Work out the finished part from the listing and answer in its coordinate system (mm). A direction names the side the tool comes from. Give positions to 0.01 mm unless a question says otherwise; leave off trailing zeros. Order: outer loops, then holes, each group sorted by start corner. A loop starts at its lowest first (then second) coordinate and runs counter-clockwise, first axis right, second up.
```python
from build123d import *

# Parameters (mm, degrees)
SKETCH1_W               = 50
SKETCH1_H               = 60
BOSS_EXTRUDE1_DEPTH     = 15
FILLET1_R               = 2
SKETCH2_W               = 40
SKETCH2_H               = 35
CUT_EXTRUDE1_DEPTH      = 6
SKETCH3_W               = 4
SKETCH3_H               = 14.5
CUT_EXTRUDE2_DEPTH      = 10
SKETCH4_R               = 2
CUT_EXTRUDE3_DEPTH      = 10
CUT_EXTRUDE4_DEPTH      = 5
CUT_EXTRUDE4_DEPTH_BACK = 6
SKETCH5_W               = 12
SKETCH5_H               = 6.5
SKETCH6_R               = 3.2
CUT_EXTRUDE5_DEPTH      = 8
SKETCH7_W               = 25
SKETCH7_H               = 10
CUT_EXTRUDE6_DEPTH      = 3.5
SKETCH8_W               = 51.392130936
SKETCH8_H               = 62.084358578
SKETCH8_W_2             = 45
SKETCH8_H_2             = 40
CUT_EXTRUDE7_DEPTH      = 13
SKETCH9_W               = 21
SKETCH9_H               = 9
CUT_EXTRUDE8_DEPTH      = 3
CUT_EXTRUDE9_DEPTH      = 7
FILLET2_R               = 5


with BuildPart() as part:
    # Sketch1 → Boss-Extrude1 (new body)
    with BuildSketch(Plane(origin=(0, 0, 0), x_dir=(1, 0, 0), z_dir=(0, 1, 0))):
        Rectangle(SKETCH1_W, SKETCH1_H)
    extrude(amount=BOSS_EXTRUDE1_DEPTH)

    # Fillet1
    fillet1_edges = [part.edges().sort_by_distance(p)[0] for p in [
        (25, 7.5, 30),
        (-25, 7.5, 30),
        (-25, 7.5, -30),
        (25, 7.5, -30),
    ]]
    fillet(fillet1_edges, radius=FILLET1_R)

    # Sketch2 → Cut-Extrude1 (cut)
    with BuildSketch(Plane(origin=(0, 15, 0), x_dir=(1, 0, 0), z_dir=(0, 1, 0))):
        with Locations((0, 5)):
            Rectangle(SKETCH2_W, SKETCH2_H)
    extrude(amount=-CUT_EXTRUDE1_DEPTH, mode=Mode.SUBTRACT)

    # Sketch3 → Cut-Extrude2 (cut)
    with BuildSketch(Plane(origin=(0, 9, 0), x_dir=(1, 0, 0), z_dir=(0, 1, 0))):
        with Locations((15.15, 7.35)):
            Rectangle(SKETCH3_W, SKETCH3_H)
    extrude(amount=-CUT_EXTRUDE2_DEPTH, mode=Mode.SUBTRACT)

    # Sketch4 → Cut-Extrude3 (cut)
    with BuildSketch(Plane.XZ):
        with Locations(Location((-14.251980034, -6.369003384, 0), (0, 0, 270))):
            Circle(SKETCH4_R)
    extrude(amount=-CUT_EXTRUDE3_DEPTH, mode=Mode.SUBTRACT)

    # Sketch5 → Cut-Extrude4 (cut, two sides: drawn at the far end of the back side and taken through both)
    with BuildSketch(Plane(origin=(0, 9, 0), x_dir=(1, 0, 0), z_dir=(0, 1, 0)).offset(-CUT_EXTRUDE4_DEPTH_BACK)):
        with Locations((0, -10)):
            Rectangle(SKETCH5_W, SKETCH5_H)
    extrude(amount=CUT_EXTRUDE4_DEPTH + CUT_EXTRUDE4_DEPTH_BACK, mode=Mode.SUBTRACT)

    # Sketch6 → Cut-Extrude5 (cut)
    with BuildSketch(Plane.XZ):
        with Locations(Location((0, 10, 0), (0, 0, 270))):
            Circle(SKETCH6_R)
    extrude(amount=-CUT_EXTRUDE5_DEPTH, mode=Mode.SUBTRACT)

    # Sketch7 → Cut-Extrude6 (cut)
    with BuildSketch(Plane(origin=(0, 15, 0), x_dir=(1, 0, 0), z_dir=(0, 1, 0))):
        with Locations((0, -12.5)):
            Rectangle(SKETCH7_W, SKETCH7_H)
    extrude(amount=-CUT_EXTRUDE6_DEPTH, mode=Mode.SUBTRACT)

    # Sketch8 → Cut-Extrude7 (cut)
    with BuildSketch(Plane(origin=(0, 0, 0), x_dir=(-1, 0, 0), z_dir=(0, -1, 0))):
        Rectangle(SKETCH8_W, SKETCH8_H)
        with Locations((0, 5)):
            Rectangle(SKETCH8_W_2, SKETCH8_H_2, mode=Mode.SUBTRACT)
    extrude(amount=-CUT_EXTRUDE7_DEPTH, mode=Mode.SUBTRACT)

    # Sketch9 → Cut-Extrude8 (cut)
    with BuildSketch(Plane(origin=(0, 15, 0), x_dir=(1, 0, 0), z_dir=(0, 1, 0))):
        with Locations((0, 22.5)):
            Rectangle(SKETCH9_W, SKETCH9_H)
    extrude(amount=-CUT_EXTRUDE8_DEPTH, mode=Mode.SUBTRACT)

    # Sketch10 → Cut-Extrude9 (cut)
    with BuildSketch(Plane.XZ):
        with BuildLine():
            Line((22.5, 15), (7.5, 15))
            ThreePointArc((7.5, 15), (0, 2.5), (-7.5, 15))
            Line((-7.5, 15), (-22.5, 15))
            Line((-22.5, 15), (-22.5, -25))
            Line((-22.5, -25), (22.5, -25))
            Line((22.5, -25), (22.5, 15))
        make_face()
    extrude(amount=-CUT_EXTRUDE9_DEPTH, mode=Mode.SUBTRACT)

    # Fillet2
    fillet2_edges = [part.edges().sort_by_distance(p)[0] for p in [
        (0, 7, 2.5),
    ]]
    fillet(fillet2_edges, radius=FILLET2_R)


solid = part.part
```
1. The mould has two halves that part along X. Classify faces 6 (the face through (0, 14, 30)), 7 (the face through (-24.43, 14.01, -29.4)), 8 (the face through (0, 9, -5)): pulls with the +X half, pulls with the -X half, needs draft (parallel to the pull), parting line crosses it, or undercut.
Findings below:
face 6: needs draft
face 7: pulls with the -X half
face 8: undercut
2. Given P1, Ø2, axis at y = 9.5, z = 14.5, coming from the +X side; P2, Ø1.8, axis at x = 14.5, y = 11, coming from the -Z side; P3, Ø5, axis at x = -2.5, z = 9, coming from the +Y side; P4, Ø5, axis at x = -1.5, z = 12, coming from the -Y side, each flat-ended and moving along its own axis, determine where each tip first touches the part or whether it passes through.
Findings below:
P1: stops at x = 22.5
P2: stops at z = -25
P3: stops at y = 9
P4: stops at y = 0
3. The part is cut by section D-D (y = 5). Write down the section's boundary in (x, z).
Findings below:
outline: (-8.62, 15) arc R9.5 ccw (long way) to (8.62, 15) - close; hole (-6, 6.75) - (6, 6.75) - (6, 13.25) - (-6, 13.25) - close
4. Which of the six approach directions +Z, -Z, +X, -X, +Y, -Y give full straight-line access (tool end or side, diameter ignored) to faces 1 (the face through (14, 11, 12.5)), 2 (the face through (0, 14, 17.5)), 3 (the face through (-24.43, 14.01, 29.4)), 4 (the face through (24.43, 14.01, -29.4)), 5 (the face through (-22.5, 10, -5))?
Findings below:
face 1: +Y
face 2: +Y, -Y
face 3: +Z, -X, +Y, -Y
face 4: -Z, +X, +Y, -Y
face 5: +Z, -Z, -X, -Y
5. Straight lines are drawn through the part: probe 1 along Z at (x, y) = (-8, 10); probe 2 along Z at (x, y) = (-5.5, 13.25); probe 3 along X at (y, z) = (11.25, -3). For each, find the intervals that lie inside material, in ascending order.
Findings below:
probe 1: z = -25 to -22.5, 12.5 to 15
probe 2: z = -30 to -27, 17.5 to 30
probe 3: x = -22.5 to -20, 20 to 22.5
6. The part is cut by section A-A (x = 0). Write down the section's boundary in (y, z), then the cut area to 3 significant figures.
Findings below:
outline: (0, 2.5) - (2, 2.5) arc R5 cw to (7, -2.5) - (7, -25) - (12, -25) - (12, -22.5) - (9, -22.5) - (9, 6.75) - (3, 6.75) - (3, 6.8) - (0, 6.8) - close; (0, 13.2) - (3, 13.2) - (3, 13.25) - (11.5, 13.25) - (11.5, 15) - (0, 15) - close; (13, -30) - (15, -30) - (15, -27) - (13, -27) - close; (13, 17.5) - (15, 17.5) - (15, 30) - (13, 30) - close
area: 158 mm2
7. The part is cut by section B-B (z = 11). Write down the section's boundary in (x, y), then the cut area to 3 significant figures.
Findings below:
outline: (-25, 13) - (-22.5, 13) - (-22.5, 7) - (-13.5, 7) arc R5 cw to (-8.5, 2) - (-8.5, 0) - (-3.04, 0) - (-3.04, 3) - (-6, 3) - (-6, 9) - (-20, 9) - (-20, 15) - (-25, 15) - close; (3.04, 0) - (8.5, 0) - (8.5, 2) arc R5 cw to (13.5, 7) - (22.5, 7) - (22.5, 13) - (25, 13) - (25, 15) - (20, 15) - (20, 9) - (6, 9) - (6, 3) - (3.04, 3) - close
area: 169 mm2
8. The part is cut by section C-C (x = -17). Write down the section's boundary in (y, z), then the cut area to 3 significant figures.
Findings below:
outline: (7, -25) - (13, -25) - (13, -30) - (15, -30) - (15, -22.5) - (9, -22.5) - (9, 12.5) - (15, 12.5) - (15, 30) - (13, 30) - (13, 15) - (7, 15) - close
area: 150 mm2
